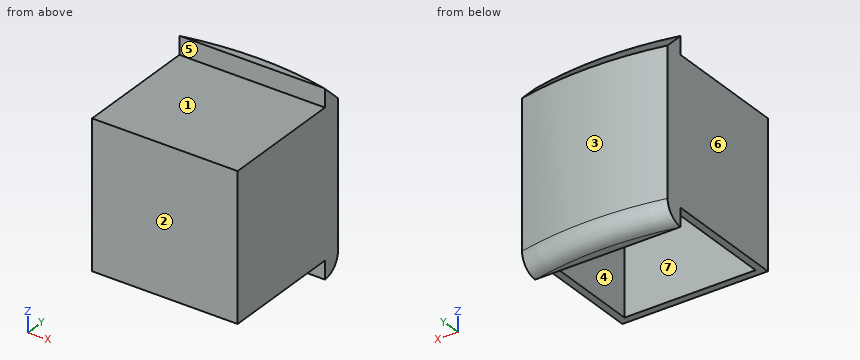
```python
from build123d import *

# Parameters (mm, degrees)
SALIENTE_EXTRUIR1_DEPTH = 50
CROQUIS4_W              = 5
CROQUIS4_H              = 34
CORTAR_EXTRUIR3_DEPTH   = 50
CROQUIS5_W              = 36
CROQUIS5_H              = 32
CORTAR_EXTRUIR4_DEPTH   = 38
REDONDEO1_R             = 5
CHAFL_N1_SIZE           = 5


with BuildPart() as part:
    # Croquis1 → Saliente-Extruir1 (new body)
    with BuildSketch(Plane.XY):
        with BuildLine():
            Line((-50.7945892, 115.897083669), (-50.7945892, 110.077719464))
            Line((-50.7945892, 110.077719464), (-50.7945892, 76.846205564))
            Line((-50.7945892, 76.846205564), (-10.7945892, 76.846205564))
            Line((-10.7945892, 76.846205564), (-10.7945892, 110.077719464))
            Line((-10.7945892, 110.077719464), (-10.7945892, 115.897083669))
            ThreePointArc((-10.7945892, 115.897083669), (-30.7945892, 118.026205564), (-50.7945892, 115.897083669))
        make_face()
    extrude(amount=SALIENTE_EXTRUIR1_DEPTH)

    # Croquis4 → Cortar-Extruir3 (cut)
    with BuildSketch(Plane.ZY.offset(50.7945892)):
        with Locations((2.5, 93.846205564)):
            Rectangle(CROQUIS4_W, CROQUIS4_H)
        with Locations((47.5, 93.846205564)):
            Rectangle(CROQUIS4_W, CROQUIS4_H)
    extrude(amount=-CORTAR_EXTRUIR3_DEPTH, mode=Mode.SUBTRACT)

    # Croquis5 → Cortar-Extruir4 (cut)
    with BuildSketch(Plane(origin=(0, 0, 5), x_dir=(-1, 0, 0), z_dir=(0, 0, -1))):
        with Locations((30.7945892, 94.846205564)):
            Rectangle(CROQUIS5_W, CROQUIS5_H)
    extrude(amount=-CORTAR_EXTRUIR4_DEPTH, mode=Mode.SUBTRACT)

    # Redondeo1
    redondeo1_edges = [part.edges().sort_by_distance(p)[0] for p in [
        (-30.7945892, 118.026205564, 0),
    ]]
    fillet(redondeo1_edges, radius=REDONDEO1_R)

    # Chaflán1
    chafl_n1_edges = [part.edges().sort_by_distance(p)[0] for p in [
        (-30.7945892, 118.026205564, 50),
    ]]
    chamfer(chafl_n1_edges, length=CHAFL_N1_SIZE)


solid = part.part
```
Part model, mm, in its own coordinate system. Face numbers are marked on the shaded views. A direction names the side the tool comes from. Round coordinates to 2 decimals unless told otherwise and drop trailing zeros. Write each loop counter-clockwise with the first axis right and the second up, starting at its lowest first coordinate (ties: lowest second). Pieces come first, ordered by that corner, then holes. Notation, with made-up numbers: (85, -29) -> (105, -29) arc R17 cw to (105, -3) -> close; hole circle Ø7 at (-18.5, -26.5). An arc over 180 degrees is marked (long way). Return JSON: item names as keys, results as strings. Group by question number.
Q1. Saw through at A-A on z = 11. Write the cut outline in (x, y).
Q2. Pin check, flat tips, straight feed: pin 1 (4 mm diameter, centred on x = -34.5, z = 47.5, fed in from -Y); pin 2 (10 mm diameter, centred on x = -33.5, y = 91.5, fed in from +Z); pin 3 (10 mm diameter, centred on x = -36, y = 87, fed in from -Z). Stop position of each tip, or through.
Q3. Saw through at B-B on y = 81. Write the cut outline in (x, z), plus the area to 3 significant figures.
Q4. Which spindle directions (+Z, -Z, +X, -X, +Y, -Y) get a long thin tool onto all of the face, cutting with end or side? Do the marked faces 5, 6 and 7. Say none if no direction does.
Q5. Mould opens along Y. For the marked faces 1, 2, 3 and 4 say: pulls with the +Y half, pulls with the -Y half, needs draft (parallel to the pull), parting line crosses it, or undercut.
Q6. Probe L1, parallel to X at y = 93.5, z = 12.5; L2, parallel to Z at x = -12.5, y = 82; L3, parallel to Z at x = -40, y = 107. List the from-to ranges inside material, lowest first. Write a range as [from, to].
Answer:
{
 "1": {"outline": "(-50.79, 76.85) -> (-10.79, 76.85) -> (-10.79, 115.9) arc R95 ccw to (-50.79, 115.9) -> close; hole (-48.79, 78.85) -> (-12.79, 78.85) -> (-12.79, 110.85) -> (-48.79, 110.85) -> close"},
 "2": {"pin 1": "y = 110.85", "pin 2": "z = 45", "pin 3": "z = 43"},
 "3": {"outline": "(-50.79, 5) -> (-48.79, 5) -> (-48.79, 43) -> (-12.79, 43) -> (-12.79, 5) -> (-10.79, 5) -> (-10.79, 45) -> (-50.79, 45) -> close", "area": "232 mm2"},
 "4": {"face 5": "+Z, +X, -X, -Y", "face 6": "+Z, -Z, -X, +Y, -Y", "face 7": "-Z"},
 "5": {"face 1": "needs draft", "face 2": "pulls with the -Y half", "face 3": "pulls with the +Y half", "face 4": "undercut"},
 "6": {"L1": "[-50.79, -48.79], [-12.79, -10.79]", "L2": "[5, 45]", "L3": "[43, 45]"}
}
